```python
from build123d import *


with BuildPart() as part:
    # Sketch1 → Revolve1 (revolve)
    with BuildSketch(Plane(origin=(0, 0, 0), x_dir=(0, 0, -1), z_dir=(1, 0, 0)), mode=Mode.PRIVATE) as revolve1_sk:
        with BuildLine():
            Line((0, 0), (0, 22.225))
            Line((0, 22.225), (89.027, 22.225))
            Line((89.027, 22.225), (89.027, 21.8186))
            Line((89.027, 21.8186), (105.029, 21.8186))
            Line((105.029, 21.8186), (105.029, 19.3675))
            ThreePointArc((105.029, 19.3675), (105.586961582, 18.020461582), (106.934, 17.4625))
            Line((106.934, 17.4625), (125.603, 17.4625))
            Line((125.603, 17.4625), (159.639, 13.4874))
            Line((159.639, 13.4874), (185.674, 13.4874))
            Line((185.674, 13.4874), (185.674, 13.2334))
            ThreePointArc((185.674, 13.2334), (185.859987194, 12.784387194), (186.309, 12.5984))
            Line((186.309, 12.5984), (188.214, 12.5984))
            Line((188.214, 12.5984), (210.058, 12.5984))
            Line((210.058, 12.5984), (210.058, 0))
            Line((210.058, 0), (0, 0))
        make_face()
    revolve(revolve1_sk.sketch.rotate(Axis((0, 0, 0), (0, 0, -1)), 90), axis=Axis((0, 0, 0), (0, 0, -1)))


solid = part.part
```
Check sheet for the modelled part. Datum: model origin and axes. Units: mm. A direction names the side the tool comes from. Coordinates: 2 decimals unless noted, no trailing zeros. Write each loop counter-clockwise with the first axis right and the second up, starting at its lowest first coordinate (ties: lowest second). Pieces come first, ordered by that corner, then holes. Notation, with made-up numbers: (56, -10.75) - (110, -10.75) arc R14 ccw to (110, 10.25) - close; hole circle Ø7 at (-34, 44). An arc over 180 degrees is marked (long way). One line per question, with ' | ' between items.
Item 1: Access from +Z, -Z, +X, -X, +Y, -Y to the whole of each face (thin tool, end or side, straight path). Record for faces 1 (the face through (0, 0, -210.058)), 2 (the face through (14.7, 16.4, -89.027)).
Determined:
face 1: -Z, +X, -X, +Y, -Y | face 2: -Z
Item 2: Sectioned sample at C-C on z = -182.5. Record the boundary of the cut face in (x, y).
Determined:
outline: circle Ø26.97 at (0, 0)
Item 3: Thickness scan on line 1 (Z direction, x = -17, y = -10); line 2 (X direction, y = -2.5, z = -174); line 3 (Z direction, x = 7.5, y = 11). Record the ranges inside material, lowest first. Write a range as [from, to].
Determined:
line 1: z = [-105.03, 0] | line 2: x = [-13.25, 13.25] | line 3: z = [-185.67, 0]
Item 4: Gauge pin test, flat ends, axial feed: P1, Ø10, axis at y = -14.5, z = -42.5, coming from the +X side; P2, Ø2, axis at y = 8, z = -41, coming from the -X side; P3, Ø1.5, axis at x = 10, z = -57.5, coming from the -Y side. Record the tip position at first contact, or that the pin passes through.
Determined:
P1: stops at x = 20.09 | P2: stops at x = -21.09 | P3: stops at y = -20.21
